```python
from build123d import *

# Parameters (mm, degrees)
F0_W     = 63.5
F0_H     = 52.5
F1_DEPTH = 4
F2_W     = 3
F2_H     = 5
F3_DEPTH = 3
F4_DEPTH = 4


with BuildPart() as f1:
    # F0 (on Top) → F1 (new body)
    with BuildSketch(Plane.XY):
        with Locations((31.75, 26.25)):
            Rectangle(F0_W, F0_H)
    extrude(amount=F1_DEPTH)

    # F2 (on face) → F3 (cut)
    with BuildSketch(Plane.XY.offset(4)):
        with Locations((13.5, 2.5)):
            Rectangle(F2_W, F2_H)
        with Locations((49, 2.5)):
            Rectangle(F2_W, F2_H)
    extrude(amount=-F3_DEPTH, mode=Mode.SUBTRACT)

    # F2 (on face) → F4 (cut)
    with BuildSketch(Plane.XY.offset(4)):
        Polygon((11, 45.5), (11, 5), (12, 5), (15, 5), (47.5, 5), (50.5, 5), (51.5, 5), (51.5, 45.5), align=None)
    extrude(amount=-F4_DEPTH, mode=Mode.SUBTRACT)


solid = f1.part
```
Input: part model. Units: mm. Frame: model coordinates. A direction names the side the tool comes from. Coordinates: 2 decimals unless noted, no trailing zeros. Write each loop counter-clockwise with the first axis right and the second up, starting at its lowest first coordinate (ties: lowest second). Pieces come first, ordered by that corner, then holes. Notation, with made-up numbers: (-23, 86.25) - (35, 86.25) arc R15 cw to (35, 111.25) - close; hole circle Ø6 at (46.25, -21.75). An arc over 180 degrees is marked (long way). Put each result on its own line as item: value. Start each with the question number.
1) Cut plane C-C (z = 3.35). Return the cut outline in (x, y).
2) Cut plane A-A (x = 13). Return the cut outline in (y, z).
3) Contact query for a flat-ended pin moving along its axis: pin 1 (1.5 mm diameter, centred on x = 49.5, y = 1.5, fed in from +Z). Output: stop coordinate, or through.
4) Ray query, L1, parallel to X at y = 30, z = 1.25; L2, parallel to Y at x = 35, z = 1.95. Return the intervals inside material, ascending.
5) Cut plane B-B (y = 6.5). Return the cut outline in (x, z).
6) Mould query, pull axis X, two halves, no side actions, for faces 1 (the face through (31, 50, 4)), 2 (the face through (32, 45.5, 2)), 3 (the face through (0, 26, 2)). Classes: pulls with the +X half, pulls with the -X half, needs draft (parallel to the pull), parting line crosses it, or undercut.
7) Reachability of faces 4 (the face through (31, 52.5, 2)), 5 (the face through (11, 26, 2)), 6 (the face through (47.5, 2, 3)) from +Z, -Z, +X, -X, +Y, -Y: full face, straight path, thin tool, end or side. Return the list, or none.
Resolved:
1. outline: (0, 0) - (12, 0) - (12, 5) - (11, 5) - (11, 45.5) - (51.5, 45.5) - (51.5, 5) - (50.5, 5) - (50.5, 0) - (63.5, 0) - (63.5, 52.5) - (0, 52.5) - close; (15, 0) - (47.5, 0) - (47.5, 5) - (15, 5) - close
2. outline: (0, 0) - (5, 0) - (5, 1) - (0, 1) - close; (45.5, 0) - (52.5, 0) - (52.5, 4) - (45.5, 4) - close
3. pin 1: stops at z = 1
4. L1: x = 0 to 11, 51.5 to 63.5
4. L2: y = 0 to 5, 45.5 to 52.5
5. outline: (0, 0) - (11, 0) - (11, 4) - (0, 4) - close; (51.5, 0) - (63.5, 0) - (63.5, 4) - (51.5, 4) - close
6. face 1: needs draft
6. face 2: undercut
6. face 3: pulls with the -X half
7. face 4: +Z, -Z, +X, -X, +Y
7. face 5: +Z, -Z
7. face 6: +Z, -Y
